For this review, take the finished solid that the model builds, in its own axes (mm). A direction names the side the tool comes from. Coordinates: 2 decimals unless noted, no trailing zeros. Loops run counter-clockwise (first coordinate to the right, second up) from the corner with the lowest first, then second, coordinate; pieces in that order, holes last. Notation, with made-up numbers: M 62,10.5 L 108,10.5 A16 ccw 108,28.5 Z; hole C 29,55 d10. An arc over 180 degrees is marked long. Write item = value, one per line.
from build123d import *

# Parameters (mm, degrees)
CUT_EXTRUDE_1_DEPTH = 2
FILLET_1_R          = 0.3
CHAMFER_1_SIZE      = 1


with BuildPart() as part:
    # Эскиз1 → Повернуть1 (revolve)
    with BuildSketch(Plane.XY):
        with BuildLine():
            Line((0, 0), (0, 4))
            ThreePointArc((0, 4), (1.41886117, 4.74341649), (3, 5))
            Line((3, 5), (3.5, 5))
            Line((3.5, 5), (3.5, 3))
            Line((3.5, 3), (15.5, 3))
            Line((15.5, 3), (15.5, 0))
            Line((15.5, 0), (0, 0))
        make_face()
    revolve(axis=Axis((15.5, 0, 0), (-1, 0, 0)))

    # Эскиз2 → Вырез-Вытянуть1 (cut)
    with BuildSketch(Plane.ZY):
        Polygon((1.154700538, 2), (-1.154700538, 2), (-2.309401077, 0), (-1.154700538, -2), (1.154700538, -2), (2.309401077, 0), align=None)
    extrude(amount=-CUT_EXTRUDE_1_DEPTH, mode=Mode.SUBTRACT)

    # Скругление1
    fillet_1_edges = [part.edges().sort_by_distance(p)[0] for p in [
        (3.5, -3, 0),
        (3.5, -5, 0),
    ]]
    fillet(fillet_1_edges, radius=FILLET_1_R)

    # Фаска1
    chamfer_1_edges = [part.edges().sort_by_distance(p)[0] for p in [
        (15.5, -3, 0),
    ]]
    chamfer(chamfer_1_edges, length=CHAMFER_1_SIZE)


solid = part.part
Q1. Draft analysis for pull direction Y (two halves, no side actions). For faces 1 (the face through (9, -3, 0)), 2 (the face through (0.99, 0.99, 1.74)), 3 (the face through (15.5, 0, 0)), state which applies: +Y half, -Y half, draft (parallel to the pull), parting line (faces both ways), or undercut.
Solved:
face_1 = parting line
face_2 = undercut
face_3 = draft
Q2. Machinability: for faces 4 (the face through (1, -2, 0)), 5 (the face through (0, -1, -2)), 6 (the face through (3.5, 2, 3)), which of the approach directions +Z, -Z, +X, -X, +Y, -Y give a long, thin tool a straight path to every point of the face, cutting with its end or side? Answer none if there is none.
Solved:
face_4 = -X
face_5 = +Z, -Z, -X, +Y, -Y
face_6 = +X
Q3. For pin 1 Ø4 at (x, y) = (4, -1.5) entering from -Z; pin 2 Ø4 at (x, z) = (4, -3) entering from -Y; pin 3 Ø2 at (x, z) = (1, -0.5) entering from +Y; pin 4 Ø1 at (x, z) = (1, 0) entering from -Y, all flat-tipped, find the tip position at first contact; note any pin that passes through.
Solved:
pin_1 = -5
pin_2 = -4.86
pin_3 = 4.89
pin_4 = -4.77
Q4. Add section B-B (x = 4). Write out the cut boundary in (y, z).
Solved:
outline = C 0,0 d6
Q5. Add section A-A (z = 0). Write out the cut boundary in (x, y).
Solved:
outline = M 0,-4 A5 ccw 3,-5 L 3.2,-5 A0.3 ccw 3.5,-4.7 L 3.5,-3.3 A0.3 cw 3.8,-3 L 14.5,-3 L 15.5,-2 L 15.5,2 L 14.5,3 L 3.8,3 A0.3 cw 3.5,3.3 L 3.5,4.7 A0.3 ccw 3.2,5 L 3,5 A5 ccw 0,4 L 0,2 L 2,2 L 2,-2 L 0,-2 Z
Q6. For line 1 along X through (y, z) = (3, 2.25); line 2 along X through (y, z) = (0, 2.5); line 3 along Y through (x, z) = (1, -1.75), list the stretches that pass through material, from the lowest coordinate up.
Solved:
line_1 = 0 to 3.5
line_2 = 0 to 15
line_3 = -4.24 to -0.97, 0.97 to 4.24
